Part model, mm, in its own coordinate system. A direction names the side the tool comes from. Give positions to 0.01 mm unless a question says otherwise; leave off trailing zeros. Loops run counter-clockwise (first coordinate to the right, second up) from the corner with the lowest first, then second, coordinate; pieces in that order, holes last. Notation, with made-up numbers: (14.5, 51) -> (54.5, 51) arc R15 cw to (54.5, 80) -> close; hole circle Ø7 at (77.25, 0). An arc over 180 degrees is marked (long way). Write item = value, one per line.
from build123d import *

# Parameters (mm, degrees)
F0_R     = 48
F1_DEPTH = 3
F3_DEPTH = 5
F5_DEPTH = 10
F6_R     = 43
F7_DEPTH = 2
F8_R     = 1


with BuildPart() as f1:
    # F0 (on Top) → F1 (new body)
    with BuildSketch(Plane.XY):
        with Locations((0.272178, 0.272177)):
            Circle(F0_R)
    extrude(amount=F1_DEPTH)

    # F2 (on face) → F3 (join)
    with BuildSketch(Plane.XY.offset(3)):
        Polygon((-0.057956, -39.281055), (33.989413, -19.690719), (34.047369, 19.590336), (0.057956, 39.281055), (-33.989413, 19.690719), (-34.047369, -19.590336), align=None)
    extrude(amount=F3_DEPTH)

    # F4 (on face) → F5 (join)
    with BuildSketch(Plane.XY.offset(8)):
        Polygon((1.531467, -13.495673), (10.625793, -8.459971), (13.495673, 1.531467), (8.459971, 10.625793), (-1.531467, 13.495673), (-10.625793, 8.459971), (-13.495673, -1.531467), (-8.459971, -10.625793), align=None)
    extrude(amount=F5_DEPTH)

    # F6 (on face) → F7 (join)
    with BuildSketch(Plane(origin=(0, 0, 0), x_dir=(1, 0, 0), z_dir=(0, 0, -1))):
        Circle(F6_R)
    extrude(amount=F7_DEPTH)

    # F8
    f8_edges = [f1.edges().sort_by_distance(p)[0] for p in [
        (-16.965728, 29.485887, 8),
        (-34.018391, 0.050192, 8),
        (-17.052663, -29.435695, 8),
        (16.965728, -29.485887, 8),
        (34.018391, -0.050192, 8),
        (17.052663, 29.435695, 8),
        (-6.07863, 10.977822, 18),
        (-12.060733, 3.464252, 18),
        (-10.977822, -6.07863, 18),
        (-3.464252, -12.060733, 18),
        (6.07863, -10.977822, 18),
        (12.060733, -3.464252, 18),
        (10.977822, 6.07863, 18),
        (3.464252, 12.060733, 18),
        (-8.459971, -10.625793, 13),
        (1.531467, -13.495673, 13),
        (10.625793, -8.459971, 13),
        (13.495673, 1.531467, 13),
        (8.459971, 10.625793, 13),
        (-1.531467, 13.495673, 13),
        (-10.625793, 8.459971, 13),
        (-13.495673, -1.531467, 13),
        (0.057956, 39.281055, 5.5),
        (34.047369, 19.590336, 5.5),
        (33.989413, -19.690719, 5.5),
        (-0.057956, -39.281055, 5.5),
        (-34.047369, -19.590336, 5.5),
        (-33.989413, 19.690719, 5.5),
        (-47.727822, 0.272177, 3),
        (-47.727822, 0.272177, 0),
        (-43, 0, -2),
    ]]
    fillet(f8_edges, radius=F8_R)


solid = f1.part
1) Which spindle directions (+Z, -Z, +X, -X, +Y, -Y) get a long thin tool onto all of the face, cutting with end or side? Do faces 1 (the face through (12.04, -3.53, 12.44)), 2 (the face through (-6.02, 11.01, 12.44)), 3 (the face through (17.284, 29.302, 4.972)), 4 (the face through (42, 11, 0)). Say none if no direction does.
Resolved:
face_1 = +Z, +X, -Y
face_2 = +Z, -X, +Y
face_3 = +Z, +X, +Y
face_4 = -Z
2) Slice it at A-A, the plane z = 13. List the corners of the cut face in (x, y), and give its area (3 significant figures).
Resolved:
outline = (-13.38, -1.13) arc R1 ccw to (-13.3, -1.89) -> (-8.66, -10.26) arc R1 ccw to (-8.06, -10.74) -> (1.13, -13.38) arc R1 ccw to (1.89, -13.3) -> (10.26, -8.66) arc R1 ccw to (10.74, -8.06) -> (13.38, 1.13) arc R1 ccw to (13.3, 1.89) -> (8.66, 10.26) arc R1 ccw to (8.06, 10.74) -> (-1.13, 13.38) arc R1 ccw to (-1.89, 13.3) -> (-10.26, 8.66) arc R1 ccw to (-10.74, 8.06) -> close
area = 522 mm²
3) Drill centre lines: line 1 along Z through (x, y) = (36.5, 9); line 2 along Z through (x, y) = (-10.5, -42); line 3 along X through (y, z) = (-17, 4.5). Where is each one in solid material? Low to high. Write a range as [from, to].
Resolved:
line_1 = [-2, 3]
line_2 = [0, 3]
line_3 = [-34.04, 33.99]
4) Drop flat-ended pins along their axis: P1, Ø12, axis at x = 28, y = -26.5, coming from the +Z side; P2, Ø12, axis at x = 12.5, z = 4, coming from the +Y side; P3, Ø1.5, axis at x = -29.5, z = 10, coming from the +Y side; P4, Ø4, axis at x = -31, y = -36, coming from the -Z side. Give the stop position or say it passes through.
Resolved:
P1 = 8
P2 = 47.82
P3 = through
P4 = 0
